Geometry check sheet. Reference: the model listing, model coordinates, mm. Face numbers are marked on the shaded views. A direction names the side the tool comes from. Give positions to 0.01 mm unless a question says otherwise; leave off trailing zeros. Order: outer loops, then holes, each group sorted by start corner. A loop starts at its lowest first (then second) coordinate and runs counter-clockwise, first axis right, second up. Notation, with made-up numbers: M -16.5,-26 L 19.5,-26 A12 cw 19.5,-11 Z; hole C 36,87.5 d2. An arc over 180 degrees is marked long. Answer as CSV lines item,"result". Start each with the question number.
Q1. Set-up check for the marked faces 1, 2 and 3: record each of +Z, -Z, +X, -X, +Y, -Y from which the full face is reachable in a straight line by a thin tool's end or side.
Q2. Thickness scan on line 1 (X direction, y = -159.5, z = 47.5); line 2 (Y direction, x = -43.5, z = 25); line 3 (X direction, y = -687, z = 43). Record the ranges inside material, lowest first.
Q3. Section check A-A, the plane x = -27.5. Record the boundary of the cut face in (y, z).
Q4. Go/stop test with flat-tipped pins: pin 1 (15 mm diameter, centred on x = -25.5, y = 24, fed in from +Z); pin 2 (15 mm diameter, centred on x = -19.5, y = -723, fed in from -Z); pin 3 (3 mm diameter, centred on x = -22, z = 25, fed in from -Y). Record where each tip stops, or that it passes through.
```python
from build123d import *

# Parameters (mm, degrees)
F0_W      = 50
F0_H      = 50
F1_DEPTH  = 700
F3_W      = 30
F3_H      = 30
F4_DEPTH  = 40
F5_W      = 30
F5_H      = 10
F6_DEPTH  = 30
F7_W      = 700
F7_H      = 10
F8_DEPTH  = 2
F9_W      = 2
F9_H      = 700
F10_DEPTH = 5


# Not quite as in the source:
# - a pattern or mirror of a feature is missing from the dataset's text; its kind, count and spacing are read off the source's solid


with BuildPart() as f1:
    # F0 (on Front) → F1 (new body)
    with BuildSketch(Plane.XZ):
        with Locations((-25, 25)):
            Rectangle(F0_W, F0_H)
    extrude(amount=F1_DEPTH)

    # F3 (on face) → F4 (join)
    with BuildSketch(Plane.XZ.offset(700)):
        with Locations((-25, 25)):
            Rectangle(F3_W, F3_H)
    f4 = extrude(amount=F4_DEPTH)

    # F4_copies: F4 across plane
    add(f4.mirror(Plane.ZX.offset(-350)))

    # F5 (on face) → F6 (cut)
    with BuildSketch(Plane.XZ.offset(740)):
        with Locations((-25, 25)):
            Rectangle(F5_W, F5_H)
    f6 = extrude(amount=-F6_DEPTH, mode=Mode.SUBTRACT)

    # F6_copies: F6 across plane
    add(f6.mirror(Plane.ZX.offset(-350)), mode=Mode.SUBTRACT)

    # F7 (on face) → F8 (cut)
    with BuildSketch(Plane.YZ):
        with Locations((-350, 45)):
            Rectangle(F7_W, F7_H)
    extrude(amount=-F8_DEPTH, mode=Mode.SUBTRACT)

    # F9 (on face) → F10 (cut)
    with BuildSketch(Plane.XY.offset(50)):
        with Locations((-4, -350)):
            Rectangle(F9_W, F9_H)
    extrude(amount=-F10_DEPTH, mode=Mode.SUBTRACT)


solid = f1.part
```
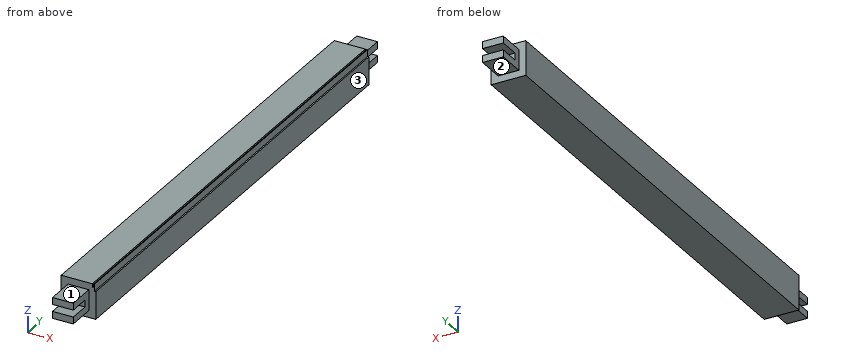
Answer block:
1,face 1,"+Z, +X, -X, -Y"
1,face 2,"-Z, +X, -X, +Y"
1,face 3,"+Z, -Z, +X, +Y, -Y"
2,line 1,"x = -50 to -5, -3 to -2"
2,line 2,"y = -700 to 0"
2,line 3,"x = -50 to -2"
3,outline,"M -740,10 L -700,10 L -700,0 L 0,0 L 0,10 L 40,10 L 40,20 L 10,20 L 10,30 L 40,30 L 40,40 L 0,40 L 0,50 L -700,50 L -700,40 L -740,40 L -740,30 L -710,30 L -710,20 L -740,20 Z"
4,pin 1,"stops at z = 40"
4,pin 2,"stops at z = 10"
4,pin 3,"stops at y = -710"
